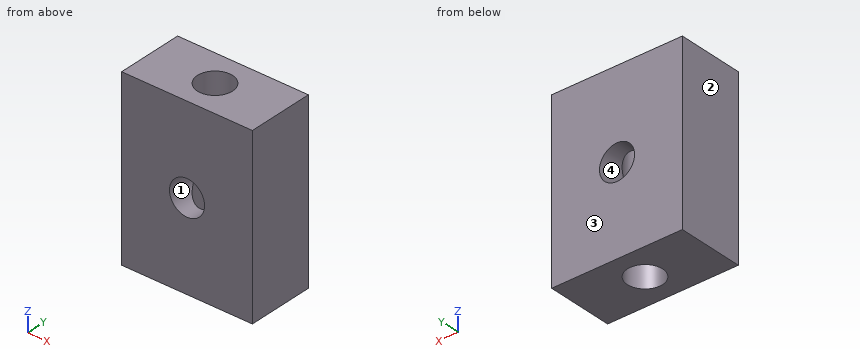
Autodesk Inventor part; units mm, degrees
ref_plane "YZ Plane" through (0, 0, 0) normal (1, 0, 0) x (0, 1, 0)
ref_plane "XZ Plane" through (0, 0, 0) normal (0, 1, 0) x (-1, 0, 0)
ref_plane "XY Plane" through (0, 0, 0) normal (0, 0, 1) x (1, 0, 0)
sketch "Sketch1" plane through (0, 0, 0) normal (0, 1, 0) x (-1, 0, 0)
  line L0 (-7.45, 10) -> (-7.45, -10)
  line L1 (-7.45, -10) -> (7.45, -10)
  line L2 (7.45, -10) -> (7.45, 10)
  line L3 (7.45, 10) -> (-7.45, 10)
  line L4 (-7.45, 10) -> (7.45, -10) construction
  line L5 (-7.45, -10) -> (7.45, 10) construction
  point P0 (0, 0)
  dimension "d0" = 14.9
  dimension "d1" = 20
extrude "Extrusion1" add sketch "Sketch1" along normal blind 7.6
sketch "Sketch2" plane through (-7.45, 0, 10) normal (0, 0, 1) x (1, 0, 0)
  line L0 (14.9, 0) -> (0, 0)
  line L1 (14.9, 7.6) -> (0, 7.6)
  line L2 (0, 0) -> (14.9, 7.6) construction
  line L3 (0, 7.6) -> (14.9, 0) construction
  circle A0 centre (7.45, 3.8) radius 2
  point P0 (7.45, 0)
  dimension "d4" = 4
extrude "Extrusion2" cut sketch "Sketch2" against normal through all
sketch "Sketch3" plane through (0, 7.6, 0) normal (0, 1, 0) x (1, 0, 0)
  circle A0 centre (0, 0) radius 2
  dimension "d7" = 4
extrude "Extrusion3" cut sketch "Sketch3" against normal through all
properties part number "MM3_track"
Here's how the part is built. I have some questions about the finished solid (model axes, mm). Face numbers are marked on the shaded views. Give positions to 0.01 mm unless a question says otherwise; leave off trailing zeros. Write each loop counter-clockwise with the first axis right and the second up, starting at its lowest first coordinate (ties: lowest second). Pieces come first, ordered by that corner, then holes. Notation, with made-up numbers: (49.25, 19.5) -> (56.25, 19.5) arc R15 cw to (56.25, 29.5) -> close; hole circle Ø9 at (-22.75, 44). An arc over 180 degrees is marked (long way). Use one line per item in the form item = value.
1) Suppose I cut it at C-C (y = 1.5). Please give me the cut outline in (x, z).
Verdict:
outline = (-7.45, -10) -> (7.45, -10) -> (7.45, 10) -> (-7.45, 10) -> close; hole circle Ø4 at (0, 0)
2) I'm going to push flat-ended pins straight in: pin 1 (3 mm diameter, centred on x = 0, z = 0, fed in from +Y); pin 2 (4 mm diameter, centred on x = -1, y = 5, fed in from -Z). Where does each tip first touch, or does it pass through?
Verdict:
pin_1 = through
pin_2 = -10
3) Suppose I cut it at D-D (z = 1). Please give me the cut outline in (x, y).
Verdict:
outline = (-7.45, 0) -> (-1.73, 0) -> (-1.73, 2.8) arc R2 cw to (-1.73, 4.8) -> (-1.73, 7.6) -> (-7.45, 7.6) -> close; (1.73, 0) -> (7.45, 0) -> (7.45, 7.6) -> (1.73, 7.6) -> (1.73, 4.8) arc R2 cw to (1.73, 2.8) -> close
4) If I drill on L1, parallel to X at y = 5.05, z = 0; L2, parallel to Y at x = 0, z = -8; L3, parallel to Y at x = -1.5, z = -3.25, over which ranges is the centre line in solid material (lowest first)? Write a range as [from, to].
Verdict:
L1 = [-7.45, -2], [2, 7.45]
L2 = [0, 1.8], [5.8, 7.6]
L3 = [0, 2.48], [5.12, 7.6]
5) Suppose I cut it at A-A (y = 5). Please give me the cut outline in (x, z).
Verdict:
outline = (-7.45, -10) -> (-1.6, -10) -> (-1.6, -1.2) arc R2 cw to (-1.6, 1.2) -> (-1.6, 10) -> (-7.45, 10) -> close; (1.6, -10) -> (7.45, -10) -> (7.45, 10) -> (1.6, 10) -> (1.6, 1.2) arc R2 cw to (1.6, -1.2) -> close
6) We'd pull the mould along X, two halves only. Please class the marked faces 1, 2, 3 and 4: +X half, -X half, draft (parallel to the pull), parting line (faces both ways), or undercut.
Verdict:
face_1 = undercut
face_2 = -X half
face_3 = draft
face_4 = undercut
7) Suppose I cut it at B-B (x = 0). Please give me the cut outline in (y, z).
Verdict:
outline = (0, -10) -> (1.8, -10) -> (1.8, -2) -> (0, -2) -> close; (0, 2) -> (1.8, 2) -> (1.8, 10) -> (0, 10) -> close; (5.8, -10) -> (7.6, -10) -> (7.6, -2) -> (5.8, -2) -> close; (5.8, 2) -> (7.6, 2) -> (7.6, 10) -> (5.8, 10) -> close
